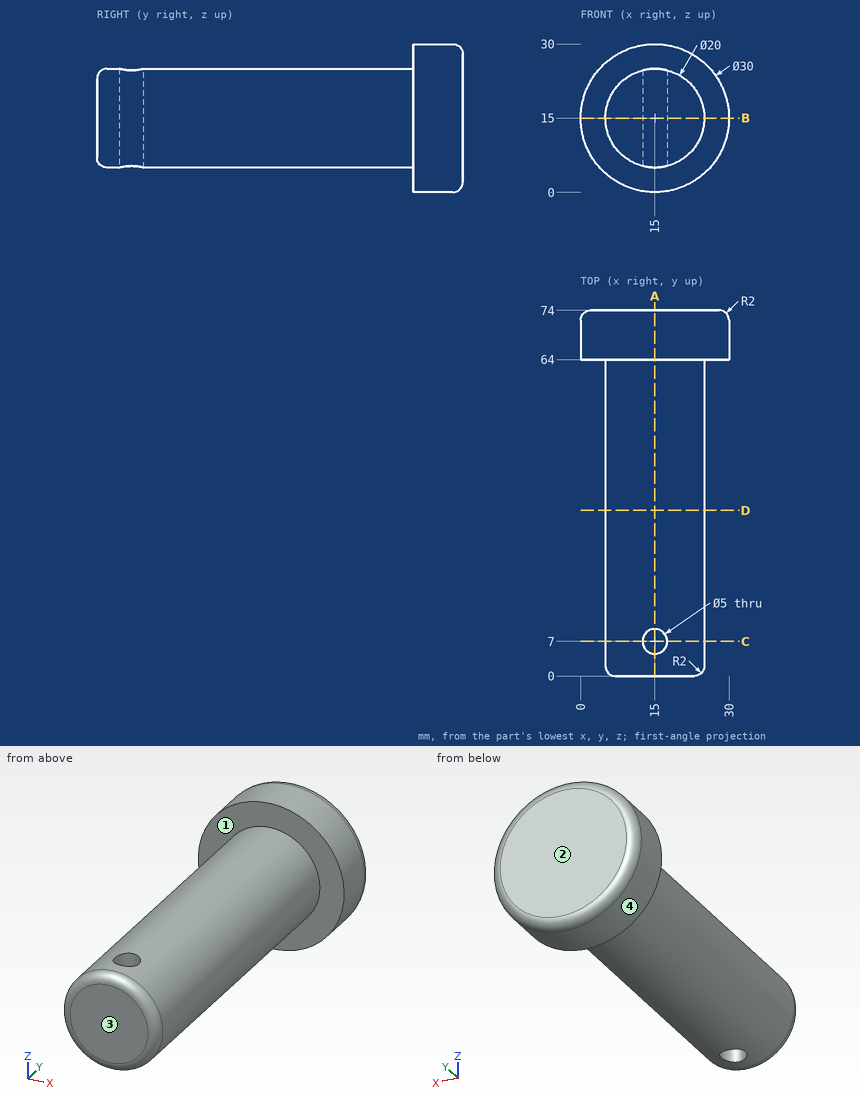
For this review, use the dimensioned drawing (mm, ordinates from the lowest corner) and the shaded views. A direction names the side the tool comes from. Give positions to 0.01 mm unless a question says otherwise; leave off trailing zeros. Loops run counter-clockwise (first coordinate to the right, second up) from the corner with the lowest first, then second, coordinate; pieces in that order, holes last.
Item 1: For line 1 along Y through (x, z) = (15, 11.25); line 2 along X through (y, z) = (65.5, 14.5); line 3 along Z through (x, y) = (14.75, 15), list the stretches that pass through material, from the lowest coordinate up.
Item 2: Take a section at A-A, the plane x = 15. State the section outline as (y, z) points.
Item 3: Insertion check: pin 1 (8 mm diameter, centred on x = 15, y = 7, fed in from -Z); pin 2 (8 mm diameter, centred on y = 15, z = 11.5, fed in from -X); pin 3 (3 mm diameter, centred on x = 10.5, y = 23, fed in from -Z). Each pin has a flat end and moves straight along its axis. Give the tip position at first contact, or say it passes through.
Item 4: Draft analysis for pull direction Z (two halves, no side actions). For the marked faces 3 and 4, state which applies: +Z half, -Z half, draft (parallel to the pull), parting line (faces both ways), or undercut.
Item 5: Take a section at B-B, the plane z = 15. State the section outline as (x, y) points.
Item 6: Take a section at D-D, the plane y = 33.5. State the section outline as (x, z) points.
Item 7: Tool access review of the marked faces 1 and 2: name each direction out of +Z, -Z, +X, -X, +Y, -Y from which nothing blocks a thin tool from reaching the whole face with its end or side.
Item 8: Take a section at C-C, the plane y = 7. State the section outline as (x, z) points, and give its area (3 significant figures).
Calculated:
1. line 1: y = 0 to 4.5, 9.5 to 74
1. line 2: x = 0.01 to 29.99
1. line 3: z = 5 to 25
2. outline: (0, 7) arc R2 ccw to (2, 5) - (4.5, 5) - (4.5, 25) - (2, 25) arc R2 ccw to (0, 23) - close; (9.5, 5) - (64, 5) - (64, 0) - (72, 0) arc R2 ccw to (74, 2) - (74, 28) arc R2 ccw to (72, 30) - (64, 30) - (64, 25) - (9.5, 25) - close
3. pin 1: stops at z = 5
3. pin 2: stops at x = 5
3. pin 3: stops at z = 5.46
4. face 3: draft
4. face 4: parting line
5. outline: (0, 64) - (5, 64) - (5, 2) arc R2 ccw to (7, 0) - (23, 0) arc R2 ccw to (25, 2) - (25, 64) - (30, 64) - (30, 72) arc R2 ccw to (28, 74) - (2, 74) arc R2 ccw to (0, 72) - close; hole circle Ø5 at (15, 7)
6. outline: circle Ø20 at (15, 15)
7. face 1: -Y
7. face 2: +Z, -Z, +X, -X, +Y
8. outline: (12.5, 5.32) - (12.5, 24.68) arc R10 ccw to start; (17.5, 5.32) arc R10 ccw to (17.5, 24.68) - close
8. area: 215 mm2
